```python
from build123d import *

# Parameters (mm, degrees)
SKETCH1_W           = 80
SKETCH1_H           = 80
BOSS_EXTRUDE1_DEPTH = 60


with BuildPart() as part:
    # Sketch1 → Boss-Extrude1 (new body)
    with BuildSketch(Plane(origin=(0, 0, 0), x_dir=(1, 0, 0), z_dir=(0, 1, 0))):
        Rectangle(SKETCH1_W, SKETCH1_H)
    extrude(amount=BOSS_EXTRUDE1_DEPTH)

    # Sketch2 → Cut-Revolve1 (revolve, cut)
    with BuildSketch(Plane.XY):
        Polygon((0, 60), (-21, 60), (-19, 58.845299462), (-17, 56.845299462), (-15, 53.381197846), (-15, 10), (0, 10), align=None)
    revolve(axis=Axis((0, 10, 0), (0, 1, 0)), mode=Mode.SUBTRACT)


solid = part.part
```
CAD build for the part. Positions are in the model's coordinates, mm. Give positions to 0.01 mm unless a question says otherwise; leave off trailing zeros. Loops run counter-clockwise (first coordinate to the right, second up) from the corner with the lowest first, then second, coordinate; pieces in that order, holes last. Notation, with made-up numbers: (55.5, 83.25) - (64.5, 83.25) arc R16 cw to (64.5, 92.25) - close; hole circle Ø8 at (50.25, -14.5). An arc over 180 degrees is marked (long way). Put each result on its own line as item: value.
Q1. Probe line 1 along Z through (x, y) = (0, 42); line 2 along Y through (x, z) = (-19, 1); line 3 along Y through (x, z) = (-13, 6). List the from-to ranges inside material, lowest first.
Filled in:
line 1: z = -40 to -15, 15 to 40
line 2: y = 0 to 58.86
line 3: y = 0 to 10
Q2. Slice it at A-A (x = 0). Give the cut face in (y, z).
Filled in:
outline: (0, -40) - (60, -40) - (60, -21) - (58.85, -19) - (56.85, -17) - (53.38, -15) - (10, -15) - (10, 15) - (53.38, 15) - (56.85, 17) - (58.85, 19) - (60, 21) - (60, 40) - (0, 40) - close
Q3. Slice it at B-B (y = 20). Give the cut face in (x, z).
Filled in:
outline: (-40, -40) - (40, -40) - (40, 40) - (-40, 40) - close; hole circle Ø30 at (0, 0)
Q4. Mould opens along Z. For faces 1 (the face through (-40, 30, 1)), 2 (the face through (14.985, 31.387, 0.66)), 3 (the face through (-1, 30, -40)), 4 (the face through (0, 10, 0)) say: pulls with the +Z half, pulls with the -Z half, needs draft (parallel to the pull), parting line crosses it, or undercut.
Filled in:
face 1: needs draft
face 2: undercut
face 3: pulls with the -Z half
face 4: undercut
Q5. Slice it at C-C (z = 0). Give the cut face in (x, y), plus the area to 3 significant figures.
Filled in:
outline: (-40, 0) - (40, 0) - (40, 60) - (21, 60) - (19, 58.85) - (17, 56.85) - (15, 53.38) - (15, 10) - (-15, 10) - (-15, 53.38) - (-17, 56.85) - (-19, 58.85) - (-21, 60) - (-40, 60) - close
area: 3,270 mm²
Q6. Flat gauge pin, fed straight in: pin 1 (9 mm diameter, centred on x = -7, z = 0.5, fed in from +Y). Where does the tip first touch, or does it go through?
Filled in:
pin 1: stops at y = 10
